Autodesk Inventor part; units mm, degrees
ref_plane "YZ Plane" through (0, 0, 0) normal (1, 0, 0) x (0, 1, 0)
ref_plane "XZ Plane" through (0, 0, 0) normal (0, 1, 0) x (-1, 0, 0)
ref_plane "XY Plane" through (0, 0, 0) normal (0, 0, 1) x (1, 0, 0)
sketch "Sketch1" plane through (0, 0, 0) normal (1, 0, 0) x (0, 1, 0)
  line L0 (0, 0) -> (70, 0)
  line L1 (70, 0) -> (70, 250)
  line L2 (70, 250) -> (0, 250)
  line L3 (0, 250) -> (0, 0)
  line L4 (70, 250) -> (30, 250)
  line L5 (30, 250) -> (30, 120)
  line L6 (30, 120) -> (70, 120)
  line L7 (70, 120) -> (70, 250)
  circle A0 centre (45, 215) radius 5
  circle A1 centre (45, 165) radius 5
  circle A2 centre (55, 82.5) radius 5
  circle A3 centre (55, 27.5) radius 5
  dimension "d0" = 70
  dimension "d1" = 250
  dimension "d2" = 50
  dimension "d3" = 10
  dimension "d4" = 25
  dimension "d5" = 130
  dimension "d6" = 40
  dimension "d7" = 35
  dimension "d12" = 10
  dimension "d13" = 15
  dimension "d14" = 55
  dimension "d15" = 27.5
extrude "Extrusion1" add sketch "Sketch1" against normal blind 24.125 contours L3 L2 L5 L6 L1 L0 | L6 L5 L2 L1 | A2 | A3
extrude "Extrusion2" cut sketch "Sketch1" against normal blind 5 contours L6 L5 L2 L1
extrude "Extrusion3" cut sketch "Sketch1" against normal through all contours A2 | A3
properties part number "bodybottompart"
Geometry: final body of the model. Coordinates: model frame, mm. A direction names the side the tool comes from. Coordinates: 2 decimals unless noted, no trailing zeros. Order: outer loops, then holes, each group sorted by start corner. A loop starts at its lowest first (then second) coordinate and runs counter-clockwise, first axis right, second up.
1) Section A-A (y = 55). Return loops of the section in (x, z) (3 decimals), then the cut area to 3 significant figures.
Result sheet:
outline: (-24.125, 0) - (0, 0) - (0, 22.5) - (-24.125, 22.5) - close; (-24.125, 32.5) - (0, 32.5) - (0, 77.5) - (-24.125, 77.5) - close; (-24.125, 87.5) - (0, 87.5) - (0, 120) - (-5, 120) - (-5, 250) - (-24.125, 250) - close
area: 4,900 mm2
2) Section C-C (x = -20.75). Return loops of the section in (y, z), then the cut area to 3 significant figures.
Result sheet:
outline: (0, 0) - (70, 0) - (70, 250) - (0, 250) - close; hole circle Ø10 at (45, 165); hole circle Ø10 at (45, 215); hole circle Ø10 at (55, 27.5); hole circle Ø10 at (55, 82.5)
area: 17,200 mm2
3) First-contact query: P1, Ø6, axis at y = 45, z = 165, coming from the +X side; P2, Ø2.5, axis at x = -3.5, z = 197, coming from the +Y side; P3, Ø8, axis at y = 61, z = 143.5, coming from the +X side. Flat tips, straight axial feed; report the tip coordinate or a pass-through.
Result sheet:
P1: passes through
P2: stops at y = 30
P3: stops at x = -5
4) Section D-D (z = 27.5). Return loops of the section in (x, y) (3 decimals).
Result sheet:
outline: (-24.125, 0) - (0, 0) - (0, 50) - (-24.125, 50) - close; (-24.125, 60) - (0, 60) - (0, 70) - (-24.125, 70) - close
5) Ray query, probe 1 along Z at (x, y) = (-12.25, 45); probe 2 along Z at (x, y) = (-13.5, 55); probe 3 along Y at (x, z) = (-10.5, 28). Return the intervals inside material, ascending.
Result sheet:
probe 1: z = 0 to 160, 170 to 210, 220 to 250
probe 2: z = 0 to 22.5, 32.5 to 77.5, 87.5 to 250
probe 3: y = 0 to 50.03, 59.97 to 70
6) Section B-B (z = 215). Return loops of the section in (x, y) (3 decimals).
Result sheet:
outline: (-24.125, 0) - (0, 0) - (0, 30) - (-5, 30) - (-5, 40) - (-24.125, 40) - close; (-24.125, 50) - (-5, 50) - (-5, 70) - (-24.125, 70) - close
7) Set-up query: faces 1 (the flat face through (-12, 70, 123)), 2 (the flat face through (-5, 50, 186)). Return all of +Z, -Z, +X, -X, +Y, -Y with unobstructed straight access to the full face (end or side cutting, diameter ignored); none if empty.
Result sheet:
face 1: +Z, -Z, +X, -X, +Y
face 2: +Z, +X, +Y
